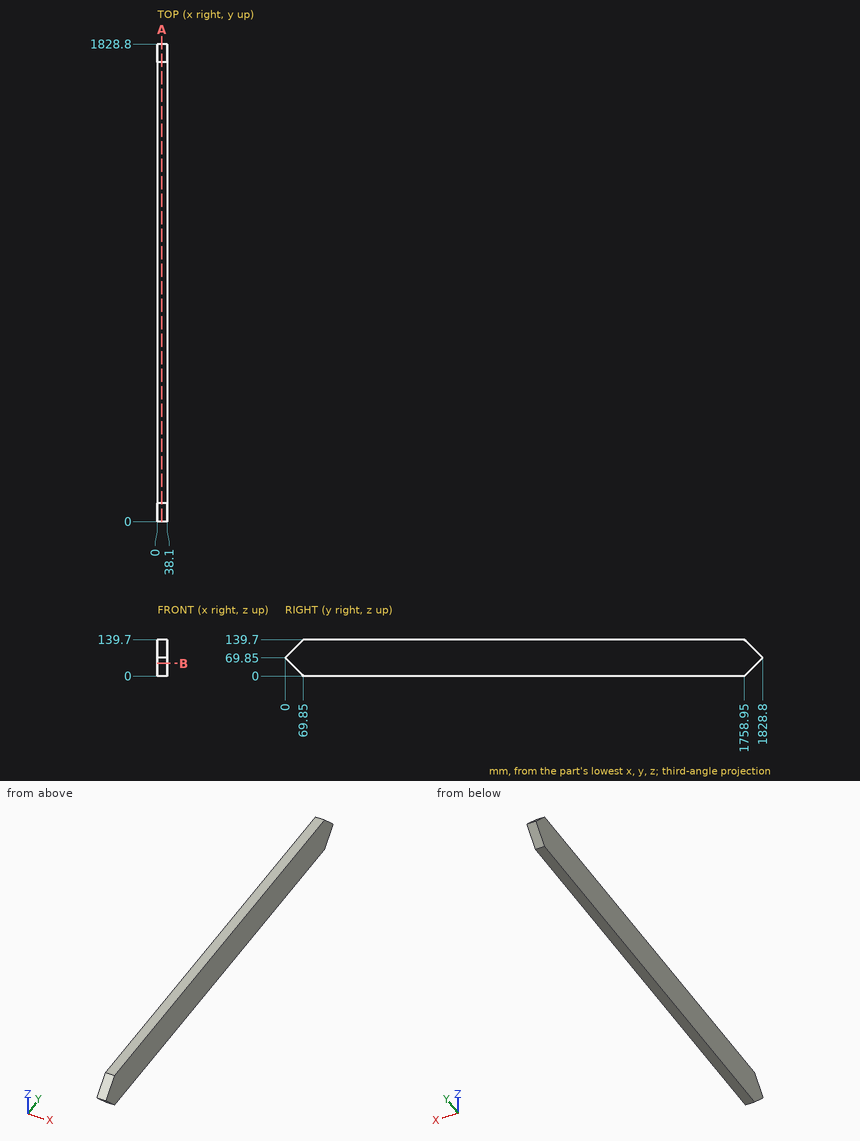
Study the drawing (mm; zero at the part's minimum x, y, z) and answer. Coordinates: 2 decimals unless noted, no trailing zeros. Order: outer loops, then holes, each group sorted by start corner. A loop starts at its lowest first (then second) coordinate and runs counter-clockwise, first axis right, second up. Notation, with made-up numbers: M 74,-25.5 L 80,-25.5 A27 cw 80,5.5 Z; hole C 50.25,60.5 d7. An arc over 180 degrees is marked long. Answer as a JSON object with one key per item and string values. Group by question number.
1. Straight lines are drawn through the part: line 1 (Y direction, x = 8, z = 42); line 2 (Y direction, x = 25.5, z = 44). For each, find the intervals that lie inside material, in ascending order.
2. Section B-B on z = 48 is taken. Write down the section's boundary in (x, y).
3. Flat-ended cylindrical pins translate along their axes: P1, Ø3, axis at x = 9.5, z = 78.5, coming from the +Y side; P2, Ø3, axis at x = 20.5, z = 87.5, coming from the -Y side. Find the tip coordinate at first contact, or state that the pin passes through.
4. Section A-A on x = 17.5 is taken. Write down the section's boundary in (y, z), then the cut area to 3 significant figures.
Values follow:
{
 "1": {"line 1": "27.85 to 1800.95", "line 2": "25.85 to 1802.95"},
 "2": {"outline": "M 0,21.85 L 38.1,21.85 L 38.1,1806.95 L 0,1806.95 Z"},
 "3": {"P1": "y = 1821.65", "P2": "y = 16.15"},
 "4": {"outline": "M 0,69.85 L 69.85,0 L 1758.95,0 L 1828.8,69.85 L 1758.95,139.7 L 69.85,139.7 Z", "area": "246,000 mm2"}
}
